The model under review builds one solid part; all positions refer to its coordinate system, in mm. Round coordinates to 2 decimals unless told otherwise and drop trailing zeros. Order: outer loops, then holes, each group sorted by start corner. A loop starts at its lowest first (then second) coordinate and runs counter-clockwise, first axis right, second up. Notation, with made-up numbers: M 17.25,-17 L 30.25,-17 A20 ccw 30.25,8 Z; hole C 19,8.25 d7. An arc over 180 degrees is marked long. Answer as a JSON object with one key per item and string values. Group by question number.
1) Consider section B-B, the plane y = -92.5. Write out the cut boundary in (x, z).
2) The part is to be moulded in two halves that separate along X. For faces 1 (the flat face through (21, 12, 3)), 2 (the cylindrical face through (-35.84, -19.61, 1.52)), say which applies: +X half, -X half, draft (parallel to the pull), parting line (faces both ways), or undercut.
3) To check wall thickness, follow line 1 (Y direction, x = 17.5, z = 0.7); line 2 (X direction, y = 98.85, z = 2) (3 decimals); line 3 (X direction, y = -100, z = 1.35). State the ranges of each line that lie inside material, in increasing order.
4) Consider section A-A, the plane x = 17.5. Write out the cut boundary in (y, z), then the cut area to 3 significant figures.
Autodesk Fusion 360 part; units mm, degrees
sketch "Sketch1" plane through (0, 0, 0) normal (0, 0, 1) x (1, 0, 0)
  line L0 (-65, 130) -> (110, 130)
  line L1 (110, 130) -> (110, -110)
  line L2 (110, -110) -> (-65, -110)
  line L3 (-65, -110) -> (-65, 130)
  dimension "d1" = 175
  dimension "d2" = 240
extrude "Extrude1" add sketch "Sketch1" along normal blind 3
sketch "Sketch2" plane through (0, 0, 3) normal (0, 0, 1) x (-1, 0, 0)
  line L0 (65, 110) -> (-110, 110)
  line L1 (-110, 110) -> (-110, -130)
  line L2 (-110, -130) -> (65, -130)
  line L3 (65, -130) -> (65, 110)
  circle A0 centre (34.5, 92.5) radius 2.5
  line L4 (60, 5.0001) -> (-105, 5)
  line L5 (12.025, 12.961) -> (3.6107, 13.032) construction
  line L6 (3.6107, 13.032) -> (3.5857, 10.071) construction
  line L7 (3.5857, 10.071) -> (12, 10) construction
  line L8 (12, 10) -> (12.025, 12.961) construction
  line L9 (-105, 5) -> (-105, 105.0001)
  line L10 (-105, 105.0001) -> (60, 105.0001)
  line L11 (12, 100) -> (-4.2428, 100.0343) construction
  line L12 (-4.2428, 100.0343) -> (-4.2609, 91.4763) construction
  line L13 (-4.2609, 91.4763) -> (11.9819, 91.4419) construction
  line L14 (11.9819, 91.4419) -> (12, 100) construction
  line L15 (60, 105.0001) -> (60, 5.0001)
  circle A1 centre (-17.5, 17.5) radius 2.5
  circle A2 centre (-17.5, 92.5) radius 2.5
  circle A3 centre (34.5, 17.5) radius 2.5
  line L16 (-46.15, -125) -> (-84, -125)
  line L17 (-84, -125) -> (-84, -97)
  line L18 (-84, -97) -> (-46.15, -97)
  line L19 (-46.15, -97) -> (-46.15, -125)
  circle A4 centre (-47.975, -123.15) radius 1
  circle A5 centre (-82.175, -123.15) radius 1
  circle A6 centre (-47.975, -98.85) radius 1
  circle A7 centre (-82.175, -98.85) radius 1
  dimension "d33" = 10
  dimension "d34" = 10
  dimension "d7" = 100
  dimension "d8" = 165
  dimension "d9" = 5
  dimension "d10" = 5
  dimension "d11" = 5
  dimension "d12" = 5
  dimension "d13" = 52
  dimension "d14" = 75
  dimension "d15" = 52
  dimension "d16" = 75
  dimension "d17" = 25.5
  dimension "d18" = 25.5
  dimension "d19" = 12.5
  dimension "d20" = 87.5
  dimension "d21" = 12.5
  dimension "d22" = 5
  dimension "d23" = 48
  dimension "d24" = 5
  dimension "d25" = 48
  dimension "d26" = 12.5
  dimension "d27" = 87.5
  dimension "d28" = 5
  dimension "d29" = 5
  dimension "d76" = 37.85
  dimension "d77" = 28
  dimension "d78" = 2
  dimension "d79" = 2
  dimension "d80" = 2
  dimension "d81" = 2
  dimension "d82" = 34.2
  dimension "d83" = 24.3
  dimension "d84" = 34.2
  dimension "d85" = 24.3
  dimension "d86" = 1.825
  dimension "d87" = 1.825
  dimension "d88" = 1.825
  dimension "d89" = 1.825
  dimension "d90" = 1.85
  dimension "d91" = 1.85
  dimension "d92" = 1.85
  dimension "d93" = 1.85
  dimension "d94" = 26
  dimension "d95" = 5
extrude "Extrude2" cut sketch "Sketch2" against normal blind 3 contours A0 | A1 | A2 | A3 | A4 | A5 | A6 | A7
sketch "Sketch3" plane through (0, 0, 3) normal (0, 0, 1) x (-1, 0, 0)
  circle A0 centre (-47.975, -123.15) radius 1
  circle A1 centre (-17.5, 92.5) radius 2.5
  circle A2 centre (34.5, 17.5) radius 2.5
  circle A3 centre (-82.175, -123.15) radius 1
  circle A4 centre (-47.975, -98.85) radius 1
  circle A5 centre (34.5, 92.5) radius 2.5
  circle A6 centre (-17.5, 17.5) radius 2.5
  circle A7 centre (-82.175, -98.85) radius 1
  line L0 (65, 110) -> (-110, 110)
  line L1 (-110, 110) -> (-110, -130)
  line L2 (-110, -130) -> (65, -130)
  line L3 (65, -130) -> (65, 110)
  circle A8 centre (55, -120) radius 1.5
  circle A9 centre (-100, -120) radius 1.5
  circle A10 centre (-100, 100) radius 1.5
  circle A11 centre (55, 100) radius 1.5
  dimension "d98" = 3
  dimension "d99" = 10
  dimension "d100" = 10
  dimension "d101" = 3
  dimension "d102" = 10
  dimension "d103" = 10
  dimension "d104" = 3
  dimension "d105" = 10
  dimension "d106" = 10
  dimension "d107" = 3
  dimension "d108" = 10
  dimension "d109" = 10
extrude "Extrude3" cut sketch "Sketch3" against normal blind 3 contours A8 | A9 | A10 | A11
Results list:
{
 "1": {"outline": "M -65,0 L -37,0 L -37,3 L -65,3 Z; M -32,0 L 15,0 L 15,3 L -32,3 Z; M 20,0 L 110,0 L 110,3 L 20,3 Z"},
 "2": {"face 1": "draft", "face 2": "undercut"},
 "3": {"line 1": "-110 to -95, -90 to -20, -15 to 130", "line 2": "-65 to 46.975, 48.975 to 81.175, 83.175 to 110", "line 3": "-65 to -56.5, -53.5 to 98.5, 101.5 to 110"},
 "4": {"outline": "M -110,0 L -95,0 L -95,3 L -110,3 Z; M -90,0 L -20,0 L -20,3 L -90,3 Z; M -15,0 L 130,0 L 130,3 L -15,3 Z", "area": "690 mm^2"}
}
